Can you work these out from the drawing? Everything is in mm from the part's minimum corner. A direction names the side the tool comes from. Give positions to 0.01 mm unless a question says otherwise; leave off trailing zeros. Loops run counter-clockwise (first coordinate to the right, second up) from the corner with the lowest first, then second, coordinate; pieces in that order, holes last. Notation, with made-up numbers: (10.25, 18) - (32.25, 18) arc R25 ccw to (32.25, 39) - close; hole circle Ø5 at (12.5, 3.25). An arc over 180 degrees is marked (long way). Answer in a Markdown table with one row per item.
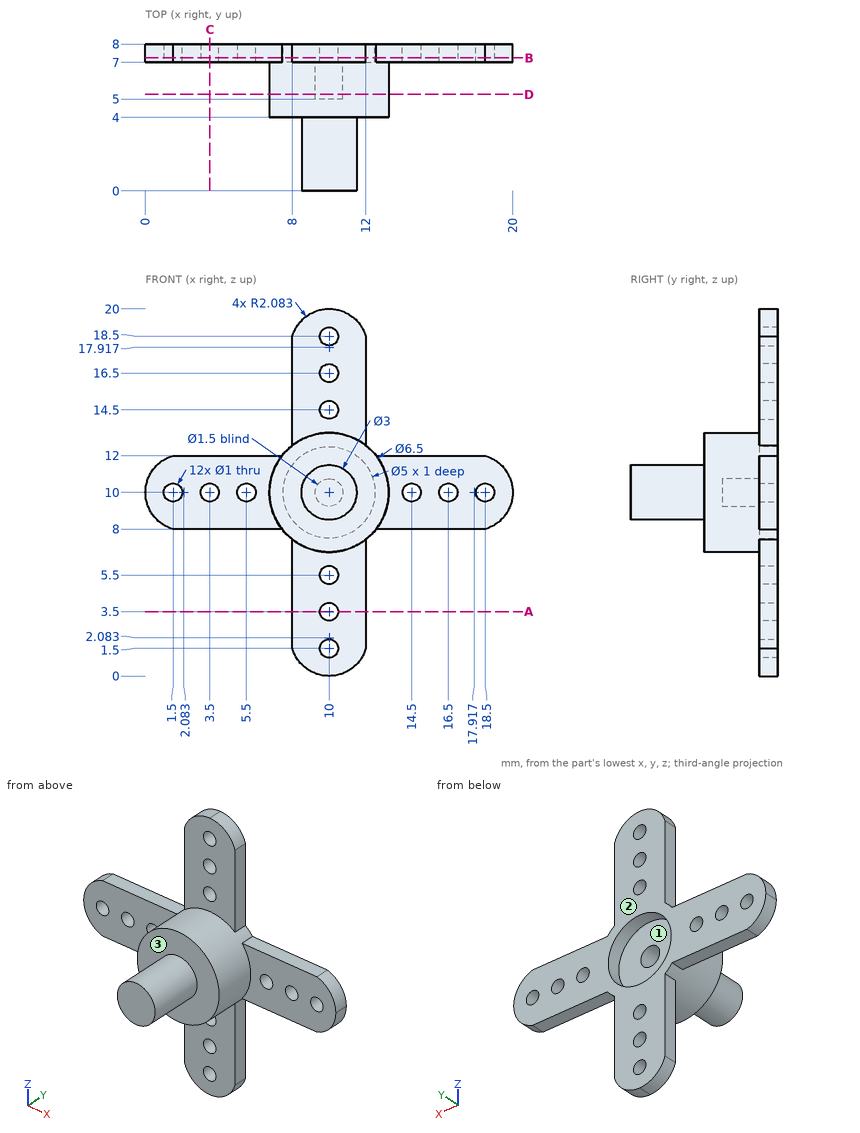
Q1. Imagine slicing it at C-C, the plane x = 3.5. Write out the boundary of the cut face in (y, z).
Checked values:
| item | result |
|---|---|
| outline | (7, 8) - (8, 8) - (8, 9.5) - (7, 9.5) - close; (7, 10.5) - (8, 10.5) - (8, 12) - (7, 12) - close |
Q2. Imagine slicing it at A-A, the plane z = 3.5. Write out the boundary of the cut face in (x, y).
Checked values:
| item | result |
|---|---|
| outline | (8, 7) - (9.5, 7) - (9.5, 8) - (8, 8) - close; (10.5, 7) - (12, 7) - (12, 8) - (10.5, 8) - close |
Q3. On a 3-axis mill with a long thin cutter (end or side, diameter ignored), from which of +Z, -Z, +X, -X, +Y, -Y can I reach the whole of each face in a straight line? I mean the marked faces 1, 2 and 3. Say none if no direction works.
Checked values:
| item | result |
|---|---|
| face 1 | +Y |
| face 2 | +Z, -Z, +X, -X, +Y |
| face 3 | -Y |
Q4. Imagine slicing it at D-D, the plane y = 5.25. Write out the boundary of the cut face in (x, z).
Checked values:
| item | result |
|---|---|
| outline | circle Ø6.5 at (10, 10); hole circle Ø1.5 at (10, 10) |
Q5. For pin 1 (0.8 mm diameter, centred on x = 16.5, y = 7.5, fed in from +Z); pin 2 (4.5 mm diameter, centred on x = 15, z = 9.5, fed in from -Y); pin 3 (1.1 mm diameter, centred on x = 15.5, y = 7.5, fed in from -Z); pin 4 (1 mm diameter, centred on x = 6, z = 6, fed in from +Y), each with a flat end and sliding along its axis, tell me the tip position at first contact or that it passes through.
Checked values:
| item | result |
|---|---|
| pin 1 | stops at z = 12 |
| pin 2 | stops at y = 4 |
| pin 3 | stops at z = 8 |
| pin 4 | passes through |
Q6. If I drill on line 1 (X direction, y = 7.3, z = 16.5); line 2 (Y direction, x = 10.75, z = 14.75), over which ranges is the centre line in solid material (lowest first)? Write a range as [from, to].
Checked values:
| item | result |
|---|---|
| line 1 | x = [8, 9.5], [10.5, 12] |
| line 2 | y = [7, 8] |
Q7. Imagine slicing it at B-B, the plane y = 7.25. Count the separate pieces of the cut face and the enclosed holes in it, and give its area (3 significant figures).
Checked values:
| item | result |
|---|---|
| separate pieces | 1 |
| enclosed holes | 13 |
| area | 109 mm² |
